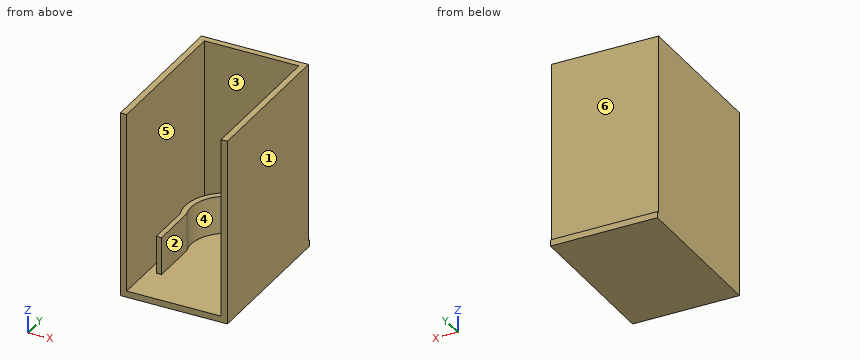
from build123d import *

# Parameters (mm, degrees)
BOSS_EXTRUDE1_DEPTH = 9
SKETCH3_W           = 22.5
SKETCH3_H           = 35
BOSS_EXTRUDE2_DEPTH = 1.5
BOSS_EXTRUDE5_DEPTH = 43
BOSS_EXTRUDE6_DEPTH = 1.5


with BuildPart() as part:
    # Sketch1 → Boss-Extrude1 (new body)
    with BuildSketch(Plane.XY):
        with BuildLine():
            Line((8, -2.872281323), (8, -14.255843504))
            Line((8, -14.255843504), (9.25, -14.255843504))
            Line((9.25, -14.255843504), (9.25, -3.491060011))
            ThreePointArc((9.25, -3.491060011), (0, 9.961709327), (-9.25, -3.491060011))
            Line((-9.25, -3.491060011), (-9.25, -14.255843504))
            Line((-9.25, -14.255843504), (-8, -14.255843504))
            Line((-8, -14.255843504), (-8, -2.872281323))
            ThreePointArc((-8, -2.872281323), (0, 8.5), (8, -2.872281323))
        make_face()
    extrude(amount=BOSS_EXTRUDE1_DEPTH)

    # Sketch3 → Boss-Extrude2 (add)
    with BuildSketch(Plane.XY):
        with Locations((0, -6.3)):
            Rectangle(SKETCH3_W, SKETCH3_H)
    extrude(amount=-BOSS_EXTRUDE2_DEPTH)



with BuildPart() as body_2:
    # Sketch9 → Boss-Extrude5 (new body)
    with BuildSketch(Plane.XY):
        Polygon((-12.75, 12.7), (12.75, 12.7), (12.75, -23.8), (11.25, -23.8), (11.25, 11.2), (-11.25, 11.2), (-11.25, -23.8), (-12.75, -23.8), align=None)
    extrude(amount=BOSS_EXTRUDE5_DEPTH)


with BuildPart() as part_1:
    add(part.part)

    add(body_2.part)  # Boss-Extrude6 merges body 2
    # Sketch10 → Boss-Extrude6 (add)
    with BuildSketch(Plane.XY):
        Polygon((-12.75, 13.2), (12.75, 13.2), (12.75, -23.8), (11.25, -23.8), (11.25, 11.2), (-11.25, 11.2), (-11.25, -23.8), (-12.75, -23.8), align=None)
    extrude(amount=-BOSS_EXTRUDE6_DEPTH)


solid = part_1.part
The listing builds one solid part. Answer for the finished solid, in the listing's coordinates (mm). Face numbers are marked on the shaded views. A direction names the side the tool comes from. Coordinates: 2 decimals unless noted, no trailing zeros. Order: outer loops, then holes, each group sorted by start corner. A loop starts at its lowest first (then second) coordinate and runs counter-clockwise, first axis right, second up.
Q1. For a pull along Y with two mould halves and no side action, classify the marked faces 4, 5 and 6 as pulls with the +Y half, pulls with the -Y half, needs draft (parallel to the pull), parting line crosses it, or undercut.
Q2. Which of the six approach directions +Z, -Z, +X, -X, +Y, -Y give full straight-line access (tool end or side, diameter ignored) to the marked faces 1, 2 and 3?
Q3. A cutting plane is placed at B-B, the plane x = 0. Write down the section's boundary in (y, z).
Q4. Consider line 1 (X direction, y = 0, z = 7); line 2 (X direction, y = 3, z = 31); line 3 (X direction, y = 3, z = 5). Determine where each line is inside the solid, lowest interval first.
Q5. A cutting plane is placed at D-D, the plane y = 1. Write down the section's boundary in (x, z).
Q6. A cutting plane is placed at C-C, the plane z = 21. Write down the section's boundary in (x, y), and give its area (3 significant figures).
Q7. Given P1, Ø1, axis at x = 8, z = 18, coming from the +Y side; P2, Ø1, axis at x = -8.5, z = 5, coming from the -Y side; P3, Ø3, axis at x = 2, z = 13.5, coming from the -Y side, each flat-ended and moving along its own axis, determine where each tip first touches the part or whether it passes through.
Q8. A cutting plane is placed at A-A, the plane z = 6.5. Write down the section's boundary in (x, y).
Answers follow:
1. face 4: undercut
1. face 5: needs draft
1. face 6: pulls with the +Y half
2. face 1: +Z, -Z, +X, +Y, -Y
2. face 2: +Z, -Y
2. face 3: +Z
3. outline: (-23.8, -1.5) - (13.2, -1.5) - (13.2, 0) - (12.7, 0) - (12.7, 43) - (11.2, 43) - (11.2, 0) - (9.96, 0) - (9.96, 9) - (8.5, 9) - (8.5, 0) - (-23.8, 0) - close
4. line 1: x = -12.75 to -11.25, -9.91 to -8.5, 8.5 to 9.91, 11.25 to 12.75
4. line 2: x = -12.75 to -11.25, 11.25 to 12.75
4. line 3: x = -12.75 to -11.25, -9.46 to -7.95, 7.95 to 9.46, 11.25 to 12.75
5. outline: (-12.75, -1.5) - (12.75, -1.5) - (12.75, 43) - (11.25, 43) - (11.25, 0) - (9.86, 0) - (9.86, 9) - (8.44, 9) - (8.44, 0) - (-8.44, 0) - (-8.44, 9) - (-9.86, 9) - (-9.86, 0) - (-11.25, 0) - (-11.25, 43) - (-12.75, 43) - close
6. outline: (-12.75, -23.8) - (-11.25, -23.8) - (-11.25, 11.2) - (11.25, 11.2) - (11.25, -23.8) - (12.75, -23.8) - (12.75, 12.7) - (-12.75, 12.7) - close
6. area: 143 mm2
7. P1: stops at y = 12.7
7. P2: stops at y = -14.26
7. P3: stops at y = 11.2
8. outline: (-12.75, -23.8) - (-11.25, -23.8) - (-11.25, 11.2) - (11.25, 11.2) - (11.25, -23.8) - (12.75, -23.8) - (12.75, 12.7) - (-12.75, 12.7) - close; (-9.25, -14.26) - (-8, -14.26) - (-8, -2.87) arc R8.5 cw (long way) to (8, -2.87) - (8, -14.26) - (9.25, -14.26) - (9.25, -3.49) arc R9.91 ccw (long way) to (-9.25, -3.49) - close
